Geometry: final body of the model. Coordinates: model frame, mm. A direction names the side the tool comes from. Round coordinates to 2 decimals unless told otherwise and drop trailing zeros. Write each loop counter-clockwise with the first axis right and the second up, starting at its lowest first coordinate (ties: lowest second). Pieces come first, ordered by that corner, then holes.
from build123d import *

# Parameters (mm, degrees)
SKETCH1_R           = 1.5
BOSS_EXTRUDE1_DEPTH = 2
SKETCH2_W           = 2.5
SKETCH2_H           = 2.5
SKETCH2_H_2         = 3
BOSS_EXTRUDE2_DEPTH = 2.5
SKETCH3_W           = 0.5
SKETCH3_H           = 0.5
BOSS_EXTRUDE3_DEPTH = 6
SKETCH4_W           = 2
SKETCH4_H           = 4
BOSS_EXTRUDE4_DEPTH = 1.5


with BuildPart() as part:
    # Sketch1 → Boss-Extrude1 (new body)
    with BuildSketch(Plane(origin=(0, 0, 0), x_dir=(1, 0, 0), z_dir=(0, 1, 0))):
        with BuildLine():
            Line((-6.5, -8), (-2.5, -8))
            Line((-2.5, -8), (-2.5, -10))
            ThreePointArc((-2.5, -10), (0, -12.5), (2.5, -10))
            Line((2.5, -10), (2.5, -8))
            Line((2.5, -8), (6.5, -8))
            Line((6.5, -8), (6.5, 8))
            Line((6.5, 8), (2.5, 8))
            Line((2.5, 8), (2.5, 10))
            ThreePointArc((2.5, 10), (0, 12.5), (-2.5, 10))
            Line((-2.5, 10), (-2.5, 8))
            Line((-2.5, 8), (-6.5, 8))
            Line((-6.5, 8), (-6.5, -8))
        make_face()
        with Locations(Location((0, 10, 0), (0, 0, 270))):
            Circle(SKETCH1_R, mode=Mode.SUBTRACT)
        with Locations(Location((0, -10, 0), (0, 0, 90))):
            Circle(SKETCH1_R, mode=Mode.SUBTRACT)
    extrude(amount=BOSS_EXTRUDE1_DEPTH)

    # Sketch2 → Boss-Extrude2 (add)
    with BuildSketch(Plane(origin=(0, 2, 0), x_dir=(1, 0, 0), z_dir=(0, 1, 0))):
        with Locations((-5.25, -6.75)):
            Rectangle(SKETCH2_W, SKETCH2_H)
        with Locations((-5.25, -4.25)):
            Rectangle(SKETCH2_W, SKETCH2_H)
        with Locations((-5.25, -1.5)):
            Rectangle(SKETCH2_W, SKETCH2_H_2)
        with Locations((-5.25, 1.5)):
            Rectangle(SKETCH2_W, SKETCH2_H_2)
        with Locations((-5.25, 4.25)):
            Rectangle(SKETCH2_W, SKETCH2_H)
        with Locations((-5.25, 6.75)):
            Rectangle(SKETCH2_W, SKETCH2_H)
    extrude(amount=BOSS_EXTRUDE2_DEPTH)

    # Sketch3 → Boss-Extrude3 (add)
    with BuildSketch(Plane(origin=(0, 4.5, 0), x_dir=(1, 0, 0), z_dir=(0, 1, 0))):
        with Locations((-5.25, -6.75)):
            Rectangle(SKETCH3_W, SKETCH3_H)
        with Locations((-5.25, -4.25)):
            Rectangle(SKETCH3_W, SKETCH3_H)
        with Locations((-5.25, -1.75)):
            Rectangle(SKETCH3_W, SKETCH3_H)
        with Locations((-5.25, 0.75)):
            Rectangle(SKETCH3_W, SKETCH3_H)
        with Locations((-5.25, 3.25)):
            Rectangle(SKETCH3_W, SKETCH3_H)
        with Locations((-5.25, 5.75)):
            Rectangle(SKETCH3_W, SKETCH3_H)
    extrude(amount=BOSS_EXTRUDE3_DEPTH)

    # Sketch4 → Boss-Extrude4 (add)
    with BuildSketch(Plane.XZ):
        with Locations((1.5, 0)):
            Rectangle(SKETCH4_W, SKETCH4_H)
    extrude(amount=BOSS_EXTRUDE4_DEPTH)


solid = part.part
1) First-contact query: P1, Ø1, axis at x = 3.5, z = 9.5, coming from the +Y side; P2, Ø6, axis at x = -2.5, y = 8.5, coming from the +Z side; P3, Ø0.6, axis at y = 6.5, z = -5.5, coming from the +X side; P4, Ø1.2, axis at x = -5.5, y = 1.5, coming from the +Z side. Flat tips, straight axial feed; report the tip coordinate or a pass-through.
2) Section B-B on y = 6.25. Output: boundary loops of the cut face in (x, z), plus the area to 3 significant figures.
3) Draft query along X for faces 1 (the cylindrical face through (-0.07, 0.99, 11.5)), 2 (the flat face through (-2.5, 1, 9)), 3 (the flat face through (2.5, 1, -9)), 4 (the flat face through (1, -1, -2)). Return one class per face: pulls with the +X half, pulls with the -X half, needs draft (parallel to the pull), parting line crosses it, or undercut.
4) Line query: probe 1 along X at (y, z) = (0.75, 10); probe 2 along Y at (x, z) = (-1.5, -5); probe 3 along X at (y, z) = (3, -2.75). Output: solid intervals per line, ascending.
5) Section A-A on x = 0. Output: boundary loops of the cut face in (y, z).
6) Reachability of faces 5 (the flat face through (5, 1, -8)), 6 (the flat face through (2.5, -1, 0)), 7 (the flat face through (-5, 2, 8)), 8 (the flat face through (4, 1, 8)) from +Z, -Z, +X, -X, +Y, -Y: full face, straight path, thin tool, end or side. Return the list, or none.
7) Section C-C on y = 0.75. Output: boundary loops of the cut face in (x, z), plus the area to 3 significant figures.
8) Section D-D on z = -2.5. Output: boundary loops of the cut face in (x, y), plus the area to 4 significant figures.
Filled in:
1. P1: passes through
1. P2: stops at z = 7
1. P3: stops at x = -5
1. P4: stops at z = 8
2. outline: (-5.5, -6) - (-5, -6) - (-5, -5.5) - (-5.5, -5.5) - close; (-5.5, -3.5) - (-5, -3.5) - (-5, -3) - (-5.5, -3) - close; (-5.5, -1) - (-5, -1) - (-5, -0.5) - (-5.5, -0.5) - close; (-5.5, 1.5) - (-5, 1.5) - (-5, 2) - (-5.5, 2) - close; (-5.5, 4) - (-5, 4) - (-5, 4.5) - (-5.5, 4.5) - close; (-5.5, 6.5) - (-5, 6.5) - (-5, 7) - (-5.5, 7) - close
2. area: 1.50 mm2
3. face 1: undercut
3. face 2: pulls with the -X half
3. face 3: pulls with the +X half
3. face 4: needs draft
4. probe 1: x = -2.5 to -1.5, 1.5 to 2.5
4. probe 2: y = 0 to 2
4. probe 3: x = -6.5 to -4
5. outline: (0, -12.5) - (2, -12.5) - (2, -11.5) - (0, -11.5) - close; (0, -8.5) - (2, -8.5) - (2, 8.5) - (0, 8.5) - close; (0, 11.5) - (2, 11.5) - (2, 12.5) - (0, 12.5) - close
6. face 5: -Z, +X, +Y, -Y
6. face 6: +Z, -Z, +X, -Y
6. face 7: +Z, -X, +Y, -Y
6. face 8: +Z, +X, +Y, -Y
7. outline: (-6.5, -8) - (-2.5, -8) - (-2.5, -10) arc R2.5 ccw to (2.5, -10) - (2.5, -8) - (6.5, -8) - (6.5, 8) - (2.5, 8) - (2.5, 10) arc R2.5 ccw to (-2.5, 10) - (-2.5, 8) - (-6.5, 8) - close; hole circle Ø3 at (0, -10); hole circle Ø3 at (0, 10)
7. area: 233 mm2
8. outline: (-6.5, 0) - (6.5, 0) - (6.5, 2) - (-4, 2) - (-4, 4.5) - (-6.5, 4.5) - close
8. area: 32.25 mm2
